For this review, take the finished solid that the model builds, in its own axes (mm). A direction names the side the tool comes from. Give positions to 0.01 mm unless a question says otherwise; leave off trailing zeros. Loops run counter-clockwise (first coordinate to the right, second up) from the corner with the lowest first, then second, coordinate; pieces in that order, holes last. Notation, with made-up numbers: M 3,57 L 37,57 A22 ccw 37,90 Z; hole C -9.5,14 d4. An arc over 180 degrees is marked long. Use CSV: the item, a comma, the result in double quotes. Start each with the question number.
1. Take a section at A-A, the plane x = -1.25. Write out the cut boundary in (y, z), and give its area (3 significant figures).
2. Take a section at B-B, the plane z = 373.5. Write out the cut boundary in (x, y).
3. Tool access review of faces 5 (the face through (11, 0, 635)), 6 (the face through (0, -9.652, -9)): name each direction out of +Z, -Z, +X, -X, +Y, -Y from which nothing blocks a thin tool from reaching the whole face with its end or side.
4. To check wall thickness, follow line 1 (Y direction, x = -6, z = -574.5). State the ranges of the line that lie inside material, in increasing order. Write a range as [from, to].
5. The part is to be moulded in two halves that separate along Y. For faces 1 (the face through (0, 12.7, -9)), 2 (the face through (9.652, 0, -9)), 3 (the face through (11, 0, -635)), 4 (the face through (-9.652, 0, -9)), say which applies: pulls with the +Y half, pulls with the -Y half, needs draft (parallel to the pull), parting line crosses it, or undercut.
6. Insertion check: P1, Ø7.5, axis at y = -3.35, z = -457.28, coming from the -X side. The pin has a flat end and moves straight along its axis. Give the tip position at first contact, or say it passes through.
Autodesk Inventor part; units mm, degrees
ref_plane "YZ Plane" through (0, 0, 0) normal (1, 0, 0) x (0, 1, 0)
ref_plane "XZ Plane" through (0, 0, 0) normal (0, 1, 0) x (-1, 0, 0)
ref_plane "XY Plane" through (0, 0, 0) normal (0, 0, 1) x (1, 0, 0)
sketch "Sketch1" plane through (0, 0, 0) normal (0, 0, 1) x (1, 0, 0)
  line L0 (-12.7, 12.7) -> (12.7, 12.7)
  line L1 (12.7, 12.7) -> (12.7, -12.7)
  line L2 (12.7, -12.7) -> (-12.7, -12.7)
  line L3 (-12.7, -12.7) -> (-12.7, 12.7)
  line L4 (9.652, 9.652) -> (-9.652, 9.652)
  line L5 (-9.652, 9.652) -> (-9.652, -9.652)
  line L6 (-9.652, -9.652) -> (9.652, -9.652)
  line L7 (9.652, -9.652) -> (9.652, 9.652)
  point P0 (0, 0)
  point P1 (0, 12.7)
  point P2 (12.7, 0)
  point P3 (-12.7, 0)
  dimension "d0" = 25.4
  dimension "d1" = 25.4
  dimension "d2" = 3.048
extrude "Extrusion1" add sketch "Sketch1" along normal mid plane 1270
sketch "Sketch2" plane through (12.7, 12.7, 635) normal (1, 0, 0) x (0, 0, -1)
  circle A0 centre (97.7242, -16.0521) radius 4.25
  circle A1 centre (177.7242, -16.0521) radius 4.25
  circle A2 centre (1092.2758, -16.0522) radius 4.25
  circle A3 centre (1172.2758, -16.0522) radius 4.25
  point P0 (635, -12.7)
hole "Hole1" at (12.7, -3.3521, 537.2758) at (12.7, -3.3521, 457.2758) at (12.7, -3.3522, -457.2758) at (12.7, -3.3522, -537.2758) direction (-1, 0, 0) diameter 6.7564 depth 12.7 tip angle 118
sketch "Sketch3" plane through (-12.7, -12.7, -635) normal (-1, 0, 0) x (0, 0, 1)
  point P0 (635, 12.7)
sketch "Sketch5" plane through (-12.7, -12.7, -635) normal (-1, 0, 0) x (0, 0, 1)
  circle A0 centre (1172.2758, 9.3479) radius 3.3782
  circle A1 centre (1092.2758, 9.3479) radius 3.3782
  circle A2 centre (1092.2758, 9.3479) radius 3.3782
  circle A3 centre (177.7242, 9.3478) radius 3.3782
  circle A4 centre (97.7242, 9.3478) radius 3.3782
  point P0 (635, 12.7)
hole "Hole2" at (-12.7, -3.3521, 537.2758) at (-12.7, -3.3521, 457.2758) at (-12.7, -3.3522, -457.2758) at (-12.7, -3.3522, -537.2758) direction (1, 0, 0) diameter 12.7 depth 3.175 tip angle 118
sketch "Sketch6" plane through (12.7, 12.7, 635) normal (1, 0, 0) x (0, 0, -1)
  circle A0 centre (1092.2758, -16.0522) radius 3.3782
  circle A1 centre (177.7242, -16.0521) radius 3.3782
  point P0 (635, -12.7)
  point P1 (298.3742, -16.0522)
  point P2 (412.6742, -16.0522)
  point P3 (857.3258, -16.0522)
  point P4 (971.6258, -16.0522)
  dimension "d19" = 120.65
  dimension "d20" = 114.3
  dimension "d21" = 120.65
  dimension "d22" = 114.3
hole "Hole3" at (12.7, -3.3522, 336.6258) at (12.7, -3.3522, 222.3258) at (12.7, -3.3522, -222.3258) at (12.7, -3.3522, -336.6258) direction (-1, 0, 0) diameter 6.7469 depth 3.175 tip angle 118
sketch "Sketch7" plane through (-12.7, -12.7, -635) normal (-1, 0, 0) x (0, 0, 1)
  circle A0 centre (971.6258, 9.3478) radius 3.3734
  circle A1 centre (857.3258, 9.3478) radius 3.3734
  circle A2 centre (412.6742, 9.3478) radius 3.3734
  circle A3 centre (298.3742, 9.3478) radius 3.3734
  circle A4 centre (971.6258, 9.3478) radius 3.3734
  line L0 (444.5, -28.493) -> (444.5, 123.907)
  line L1 (266.7, -34.843) -> (444.5, -34.843)
  line L2 (266.7, -34.843) -> (444.5, -34.843)
  line L3 (444.5, 130.257) -> (266.7, 130.257)
  point P0 (635, 12.7)
hole "Hole4" at (-12.7, -3.3522, 336.6258) at (-12.7, -3.3522, 222.3258) at (-12.7, -3.3522, -222.3258) at (-12.7, -3.3522, -336.6258) direction (1, 0, 0) diameter 12.7 depth 3.175 tip angle 118
equation "\"d2\" = thick"
equation "\"d3\" = L"
equation "\"L\" = 1270"
equation "\"thick\" = 3.048"
properties part number "1inSquareSupport2"
Result set:
1,outline,"M -12.7,-635 L -9.65,-635 L -9.65,635 L -12.7,635 Z; M 9.65,-635 L 12.7,-635 L 12.7,635 L 9.65,635 Z"
1,area,"7,740 mm2"
2,outline,"M -12.7,-12.7 L 12.7,-12.7 L 12.7,12.7 L -12.7,12.7 Z; hole M -9.65,-9.65 L 9.65,-9.65 L 9.65,9.65 L -9.65,9.65 Z"
3,face 5,"+Z, +X, -X, +Y, -Y"
3,face 6,"+Z, -Z"
4,line 1,"[-12.7, -9.65], [9.65, 12.7]"
5,face 1,"pulls with the +Y half"
5,face 2,"undercut"
5,face 3,"needs draft"
5,face 4,"undercut"
6,P1,"x = 9.65"
